Geometry: final body of the model. Coordinates: model frame, mm. Face numbers are marked on the shaded views. A direction names the side the tool comes from. Give positions to 0.01 mm unless a question says otherwise; leave off trailing zeros. Order: outer loops, then holes, each group sorted by start corner. A loop starts at its lowest first (then second) coordinate and runs counter-clockwise, first axis right, second up. Notation, with made-up numbers: (-38.5, 77.25) -> (-17.5, 77.25) arc R25 ccw to (-17.5, 101.25) -> close; hole circle Ø10 at (28.25, 88). An arc over 180 degrees is marked (long way). One line per question, with ' | ' between items. Start each with the question number.
(1) Section C-C (x = -30). Return loops of the section in (y, z).
(2) Section A-A (z = 10). Return loops of the section in (x, y).
(3) Section B-B (y = 0). Return loops of the section in (x, z), then the cut area to 3 significant figures.
(4) First-contact query: pin 1 Ø1 at (x, y) = (-25, 7) entering from -Z. Flat tip, straight axial feed; report the tip coordinate or a pass-through.
(5) Mould query, pull axis X, two halves, no side actions, for the marked faces 3, 4, 5 and 6. Classes: +X half, -X half, draft (parallel to the pull), parting line (faces both ways), or undercut.
(6) Set-up query: the marked faces 1 and 2. Return all of +Z, -Z, +X, -X, +Y, -Y with unobstructed straight access to the full face (end or side cutting, diameter ignored); none if empty.
(7) Section D-D (y = 2.75). Return loops of the section in (x, z), then the cut area to 3 significant figures.
(8) Ray query, L1, parallel to X at y = 6.75, z = -1.75; L2, parallel to Z at x = -14, y = 6.75; L3, parallel to Z at x = 1, y = -8. Return the intervals inside material, ascending.
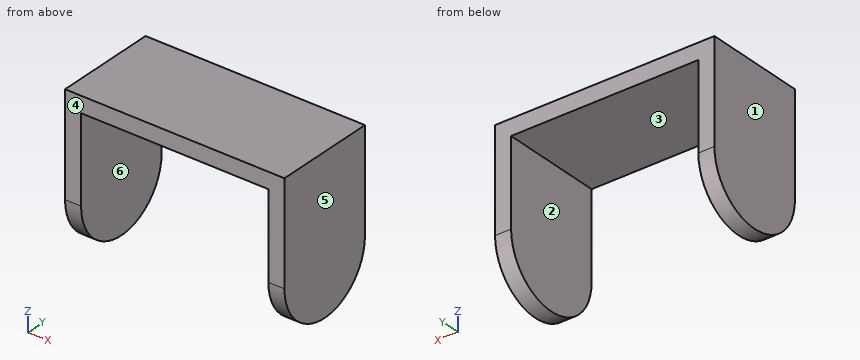
```python
from build123d import *

# Parameters (mm, degrees)
SKETCH1_R           = 9.6
SKETCH1_W           = 3
SKETCH1_H           = 19.2
BOSS_EXTRUDE1_DEPTH = 3
SKETCH1_3_W         = 3
SKETCH1_3_H         = 19.2
BOSS_EXTRUDE2_DEPTH = 38
BOSS_EXTRUDE3_START = -38
SKETCH1_4_R         = 9.6
BOSS_EXTRUDE3_DEPTH = 38
CUT_EXTRUDE1_START  = -35
SKETCH1_5_R         = 9.6
CUT_EXTRUDE1_DEPTH  = 35


with BuildPart() as part:
    # Sketch1 → Boss-Extrude1 (new body)
    with BuildSketch(Plane(origin=(0, 0, 0), x_dir=(0, 0, -1), z_dir=(1, 0, 0))):
        Circle(SKETCH1_R)
        with BuildLine():
            Line((-16, -9.6), (0, -9.6))
            ThreePointArc((0, -9.6), (-9.6, 0), (0, 9.6))
            Line((0, 9.6), (-16, 9.6))
            Line((-16, 9.6), (-16, -9.6))
        make_face()
        with Locations((-17.5, 0)):
            Rectangle(SKETCH1_W, SKETCH1_H)
    extrude(amount=BOSS_EXTRUDE1_DEPTH)

    # Sketch1_3 → Boss-Extrude2 (add)
    with BuildSketch(Plane(origin=(0, 0, 0), x_dir=(0, 0, -1), z_dir=(1, 0, 0))):
        with Locations((-17.5, 0)):
            Rectangle(SKETCH1_3_W, SKETCH1_3_H)
    extrude(amount=-BOSS_EXTRUDE2_DEPTH)

    # Sketch1_4 → Boss-Extrude3 (add)
    with BuildSketch(Plane(origin=(0, 0, 0), x_dir=(0, 0, -1), z_dir=(1, 0, 0)).offset(BOSS_EXTRUDE3_START)):
        with BuildLine():
            Line((-16, -9.6), (0, -9.6))
            ThreePointArc((0, -9.6), (-9.6, 0), (0, 9.6))
            Line((0, 9.6), (-16, 9.6))
            Line((-16, 9.6), (-16, -9.6))
        make_face()
        Circle(SKETCH1_4_R)
    extrude(amount=BOSS_EXTRUDE3_DEPTH)

    # Sketch1_5 → Cut-Extrude1 (cut)
    with BuildSketch(Plane(origin=(0, 0, 0), x_dir=(0, 0, -1), z_dir=(1, 0, 0)).offset(CUT_EXTRUDE1_START)):
        Circle(SKETCH1_5_R)
        with BuildLine():
            Line((-16, -9.6), (0, -9.6))
            ThreePointArc((0, -9.6), (-9.6, 0), (0, 9.6))
            Line((0, 9.6), (-16, 9.6))
            Line((-16, 9.6), (-16, -9.6))
        make_face()
    extrude(amount=CUT_EXTRUDE1_DEPTH, mode=Mode.SUBTRACT)


solid = part.part
```
Response:
1) outline: (-9.6, 16) -> (9.6, 16) -> (9.6, 19) -> (-9.6, 19) -> close
2) outline: (-38, -9.6) -> (-35, -9.6) -> (-35, 9.6) -> (-38, 9.6) -> close; (0, -9.6) -> (3, -9.6) -> (3, 9.6) -> (0, 9.6) -> close
3) outline: (-38, -9.6) -> (-35, -9.6) -> (-35, 16) -> (0, 16) -> (0, -9.6) -> (3, -9.6) -> (3, 19) -> (-38, 19) -> close | area: 277 mm^2
4) pin 1: stops at z = 16
5) face 3: undercut | face 4: draft | face 5: +X half | face 6: undercut
6) face 1: +Z, -Z, -X, +Y, -Y | face 2: -Z, +Y, -Y
7) outline: (-38, -9.2) -> (-35, -9.2) -> (-35, 16) -> (0, 16) -> (0, -9.2) -> (3, -9.2) -> (3, 19) -> (-38, 19) -> close | area: 274 mm^2
8) L1: x = -38 to -35, 0 to 3 | L2: z = 16 to 19 | L3: z = -5.31 to 19
